Design review of the part shown in the three views and the two pictorial views. Dimensions are in mm from the part's minimum x, y and z. A direction names the side the tool comes from. Give positions to 0.01 mm unless a question says otherwise; leave off trailing zeros. Order: outer loops, then holes, each group sorted by start corner. A loop starts at its lowest first (then second) coordinate and runs counter-clockwise, first axis right, second up.
Item 1: Machinability: for the marked faces 4 and 5, which of the approach directions +Z, -Z, +X, -X, +Y, -Y give a long, thin tool a straight path to every point of the face, cutting with its end or side? Answer none if there is none.
Item 2: For probe 1 along X at (y, z) = (19, 20); probe 2 along Y at (x, z) = (35.5, 29); probe 3 along X at (y, z) = (3.5, 27.5), list the stretches that pass through material, from the lowest coordinate up.
Item 3: Consider section A-A (y = 24). Give the boundary of the cut face in (x, z), plus the area to 3 significant figures.
Item 4: Consider section C-C (x = 23). Give the boundary of the cut face in (y, z), plus the area to 3 significant figures.
Item 5: The part is to be moulded in two halves that separate along X. For the marked faces 1, 2 and 3, say which applies: released by +X, released by -X, zero draft, split by the parting line, or undercut.
Item 6: For P1, Ø8, axis at x = 19, z = 33.5, coming from the -Y side; P2, Ø1, axis at y = 26, z = 11.5, coming from the +X side, all flat-tipped, find the tip position at first contact; note any pin that passes through.
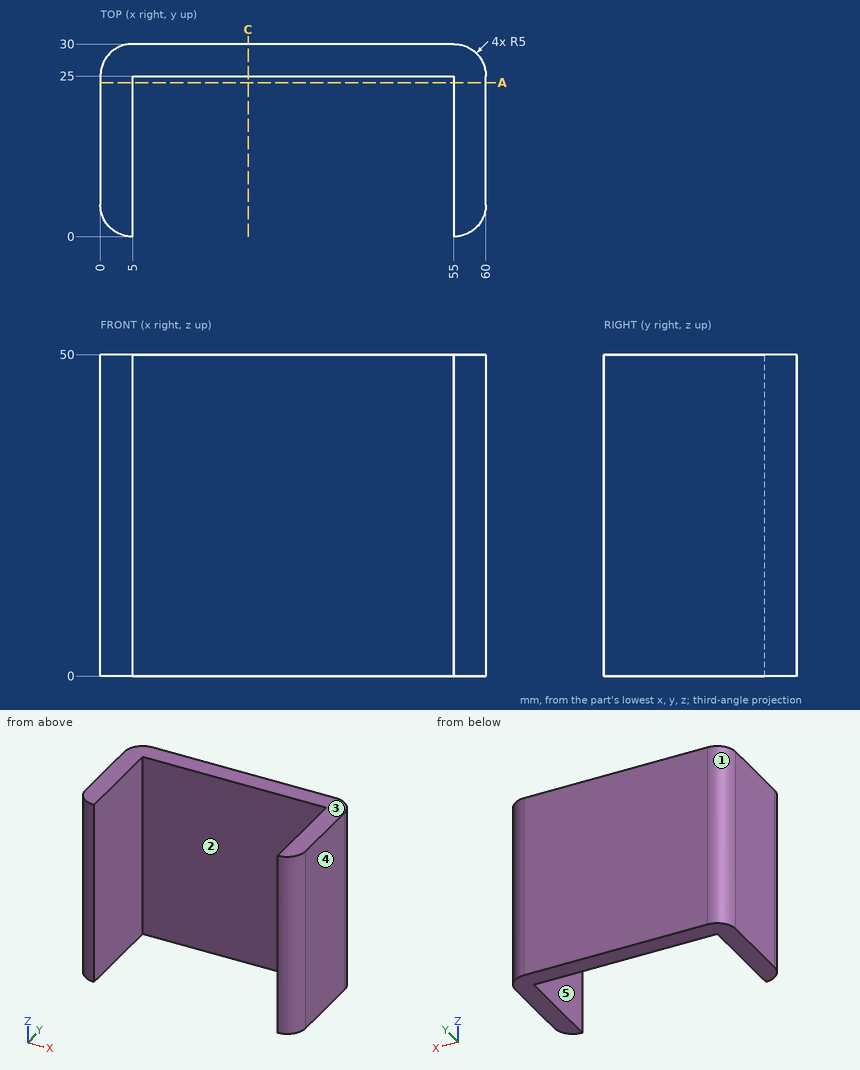
Resolved:
1. face 4: +Z, -Z, +X, +Y, -Y
1. face 5: +Z, -Z, -Y
2. probe 1: x = 0 to 5, 55 to 60
2. probe 2: y = 25 to 30
2. probe 3: x = 0.23 to 5, 55 to 59.77
3. outline: (0, 0) - (5, 0) - (5, 50) - (0, 50) - close; (55, 0) - (60, 0) - (60, 50) - (55, 50) - close
3. area: 500 mm2
4. outline: (25, 0) - (30, 0) - (30, 50) - (25, 50) - close
4. area: 250 mm2
5. face 1: released by -X
5. face 2: undercut
5. face 3: zero draft
6. P1: stops at y = 25
6. P2: stops at x = 59.97
